from build123d import *

# Parameters (mm, degrees)
ESQUISSE2_R             = 2
ENL_V_MAT_EXTRU_1_DEPTH = 23.134437673


with BuildPart() as part:
    # Esquisse1 → Révolution1 (revolve)
    with BuildSketch(Plane.XY, mode=Mode.PRIVATE) as r_volution1_sk:
        Polygon((-2.495, -19.585017995), (-2.495, 0), (-4.146462722, 0), (-4, 17.466969529), (-7.292475615, 17.466969529), (-7.292475615, -19.585017995), align=None)
    revolve(r_volution1_sk.sketch.rotate(Axis((0, 0, 0), (0, -1, 0)), 270), axis=Axis((0, 0, 0), (0, -1, 0)))

    # Esquisse2 → Enlèv. mat.-Extru.1 (cut, through all)
    with BuildSketch(Plane.XY):
        with Locations(Location((0, 8.733484764, 0), (0, 0, 90))):
            Circle(ESQUISSE2_R)
        with Locations((0, -9.792508998)):
            Circle(ESQUISSE2_R)
    extrude(amount=-ENL_V_MAT_EXTRU_1_DEPTH, mode=Mode.SUBTRACT)


solid = part.part
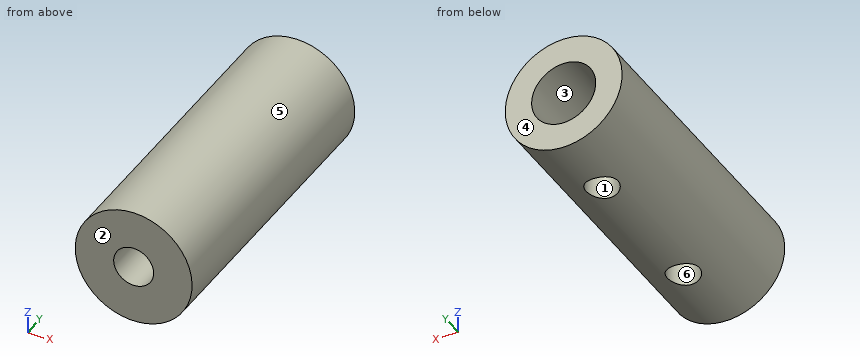
The model under review builds one solid part; all positions refer to its coordinate system, in mm. Face numbers are marked on the shaded views. A direction names the side the tool comes from. Give positions to 0.01 mm unless a question says otherwise; leave off trailing zeros. Order: outer loops, then holes, each group sorted by start corner. A loop starts at its lowest first (then second) coordinate and runs counter-clockwise, first axis right, second up. Notation, with made-up numbers: M 48.25,56.5 L 73.25,56.5 A28 cw 73.25,83.5 Z; hole C 52,-9.5 d10. An arc over 180 degrees is marked long. Answer in a Markdown table with one row per item. Add a question column.
1. Add section C-C on x = 6. State the section outline as (y, z) points.
2. Add section B-B on x = 0. Count the separate pieces of the cut face and the enclosed holes in it, plus the area to 3 significant figures.
3. Machinability: for the marked faces 1, 2 and 3, which of the approach directions +Z, -Z, +X, -X, +Y, -Y give a long, thin tool a straight path to every point of the face, cutting with its end or side? Answer none if there is none.
4. Add section A-A on y = -15. State the section outline as (x, z) points (3 decimals).
5. Mouldability with a two-part tool opening along X and no side actions: class the marked faces 4, 5 and 6 as released by +X, released by -X, zero draft, split by the parting line, or undercut.
6. To check wall thickness, follow line 1 along Y through (x, z) = (0, -3.6); line 2 along X through (y, z) = (-8.25, 0) (3 decimals); line 3 along X through (y, z) = (9.5, -4.75). State the ranges of each line that lie inside material, in increasing order.
7. Add section D-D on y = -10.5. State the section outline as (x, z) points (3 decimals), plus the area to 3 significant figures.
8. For pin 1 Ø2 at (x, y) = (-4, -1) entering from +Z; pin 2 Ø3 at (y, z) = (-0.5, -2) entering from -X; pin 3 Ø1 at (x, y) = (1, -0.5) entering from +Z, all flat-tipped, find the tip position at first contact; note any pin that passes through.
The answers:
| question | item | result |
|---|---|---|
| 1 | outline | M -19.59,-4.14 L 17.47,-4.14 L 17.47,4.14 L -19.59,4.14 Z |
| 2 | separate pieces | 4 |
| 2 | enclosed holes | 0 |
| 2 | area | 268 mm2 |
| 3 | face 1 | -Z |
| 3 | face 2 | +Z, -Z, +X, -X, -Y |
| 3 | face 3 | none |
| 4 | outline | C 0,0 d14.585; hole C 0,0 d4.99 |
| 5 | face 4 | zero draft |
| 5 | face 5 | split by the parting line |
| 5 | face 6 | undercut |
| 6 | line 1 | -19.59 to -11.79, -7.79 to 0 |
| 6 | line 2 | -7.292 to -2.495, 2.495 to 7.292 |
| 6 | line 3 | -5.53 to -1.85, 1.85 to 5.53 |
| 7 | outline | M -1.871,-7.048 L -1.871,-1.651 A2.495 cw long 1.871,-1.651 L 1.871,-7.048 A7.292 ccw long Z |
| 7 | area | 129 mm2 |
| 8 | pin 1 | z = 6.65 |
| 8 | pin 2 | x = -7.28 |
| 8 | pin 3 | z = 7.28 |
